Can you work these out from the drawing? Everything is in mm from the part's minimum corner. Give positions to 0.01 mm unless a question says otherwise; leave off trailing zeros. Order: outer loops, then holes, each group sorted by start corner. A loop starts at its lowest first (then second) coordinate and runs counter-clockwise, first axis right, second up. Notation, with made-up numbers: (62, 37) -> (70, 37) arc R25 cw to (70, 74) -> close; hole circle Ø1 at (10.5, 2.25). An arc over 180 degrees is marked (long way). Answer as CSV lines item,"result". Start each with the question number.
(1) I need wall thicknesses on L1, parallel to Y at x = 4.75, z = 25.75 (1 decimal); L2, parallel to Z at x = 5.5, y = 4 (1 decimal); L3, parallel to Z at x = 0.5, y = 3. Which ranges of each line are inside material? Lowest first, please.
(2) Will these pins go through, and if not, where does the flat tip stop? pin 1 Ø3 at (y, z) = (8, 4.5) entering from +X; pin 2 Ø3 at (y, z) = (6, 14.5) entering from +X (1 decimal); pin 3 Ø2 at (x, z) = (6.5, 15) entering from +Y; pin 4 Ø1.5 at (y, z) = (2.5, 8) entering from -X.
(3) We'd pull the mould along Y, two halves only. Please class the marked faces 1, 2 and 3: released by +Y, released by -Y, zero draft, split by the parting line, or undercut.
(4) I want a section at C-C (z = 25). Please give me the cut outline in (x, y) (1 decimal), plus the area to 3 significant figures.
(5) I want a section at B-B (y = 2.5). Please give me the cut outline in (x, z).
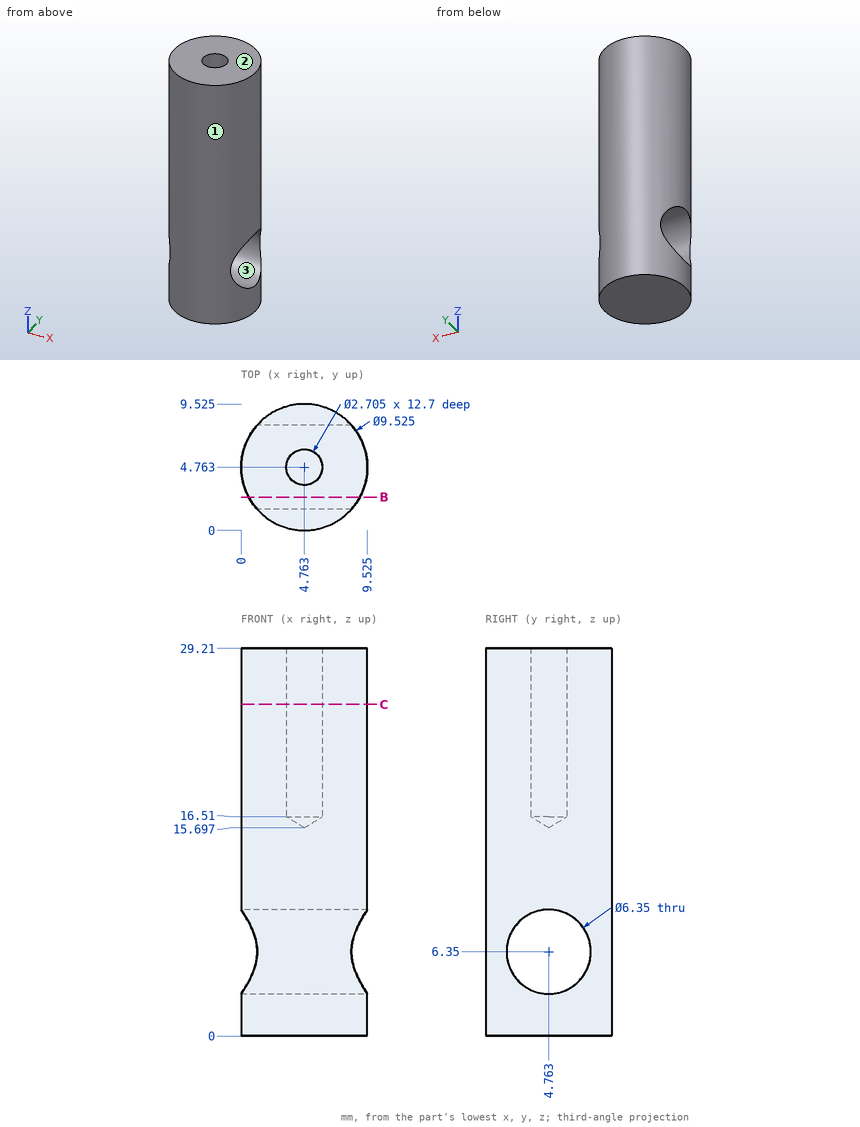
Final values:
1,L1,"0 to 3.4, 6.1 to 9.5"
1,L2,"0 to 3.3, 9.4 to 16.3"
1,L3,"0 to 3.71, 8.99 to 29.21"
2,pin 1,"x = 9.13"
2,pin 2,"x = 9.5"
2,pin 3,"y = 9.47"
2,pin 4,"x = 0.49"
3,face 1,"split by the parting line"
3,face 2,"zero draft"
3,face 3,"undercut"
4,outline,"circle Ø9.5 at (4.8, 4.8); hole circle Ø2.7 at (4.8, 4.8)"
4,area,"65.5 mm²"
5,outline,"(0.57, 0) -> (8.95, 0) -> (8.95, 4.12) -> (0.57, 4.12) -> close; (0.57, 8.58) -> (8.95, 8.58) -> (8.95, 29.21) -> (0.57, 29.21) -> close"
